from build123d import *

# Parameters (mm, degrees)
CUT_EXTRUDE_1_REACH = 23.089
SKETCH_7_R          = 1.5
CUT_EXTRUDE_2_DEPTH = 16
CUT_EXTRUDE_3_REACH = 23.089
SKETCH_8_R          = 1.5


with BuildPart() as part:
    # 草图4 → 旋转1 (revolve)
    with BuildSketch(Plane.XY, mode=Mode.PRIVATE) as revolve_1_sk:
        Polygon((0, 0), (0, 12.5), (4, 12.5), (4, 5.5), (11.5, 5.5), (11.5, 0), align=None)
    revolve(revolve_1_sk.sketch.rotate(Axis((0, 0, 0), (1, 0, 0)), 90), axis=Axis((0, 0, 0), (1, 0, 0)))

    # 草图5 → 切除-拉伸1 (cut, up to next)
    with BuildSketch(Plane(origin=(11.5, 0, 0), x_dir=(0, 0, -1), z_dir=(1, 0, 0)), mode=Mode.PRIVATE) as cut_extrude_1_sk1:
        with BuildLine():
            Line((-1.658312395, 2.5), (1.658312395, 2.5))
            ThreePointArc((1.658312395, 2.5), (0, -3), (-1.658312395, 2.5))
        make_face()
    cut_extrude_1_tool1 = extrude(cut_extrude_1_sk1.sketch, amount=-CUT_EXTRUDE_1_REACH, mode=Mode.PRIVATE) & part.part
    add(cut_extrude_1_tool1.solids().sort_by_distance((11.5, -0.111984, 0))[0], mode=Mode.SUBTRACT)

    # 草图7 → 切除-拉伸2 (cut)
    with BuildSketch(Plane(origin=(0, 6.5, 0), x_dir=(1, 0, 0), z_dir=(0, 1, 0))):
        with Locations(Location((9, 0, 0), (0, 0, 270))):
            Circle(SKETCH_7_R)
    extrude(amount=-CUT_EXTRUDE_2_DEPTH, mode=Mode.SUBTRACT)

    # 草图8 → 切除-拉伸3 (cut, up to next)
    with BuildSketch(Plane.ZY, mode=Mode.PRIVATE) as cut_extrude_3_sk1:
        with Locations((9, 0)):
            Circle(SKETCH_8_R)
    cut_extrude_3_tool1 = extrude(cut_extrude_3_sk1.sketch, amount=-CUT_EXTRUDE_3_REACH, mode=Mode.PRIVATE) & part.part
    # 草图8 → 切除-拉伸3 (cut, up to next)
    with BuildSketch(Plane.ZY, mode=Mode.PRIVATE) as cut_extrude_3_sk2:
        with Locations((0, -9)):
            Circle(SKETCH_8_R)
    cut_extrude_3_tool2 = extrude(cut_extrude_3_sk2.sketch, amount=-CUT_EXTRUDE_3_REACH, mode=Mode.PRIVATE) & part.part
    # 草图8 → 切除-拉伸3 (cut, up to next)
    with BuildSketch(Plane.ZY, mode=Mode.PRIVATE) as cut_extrude_3_sk3:
        with Locations((-9, 0)):
            Circle(SKETCH_8_R)
    cut_extrude_3_tool3 = extrude(cut_extrude_3_sk3.sketch, amount=-CUT_EXTRUDE_3_REACH, mode=Mode.PRIVATE) & part.part
    # 草图8 → 切除-拉伸3 (cut, up to next)
    with BuildSketch(Plane.ZY, mode=Mode.PRIVATE) as cut_extrude_3_sk4:
        with Locations((0, 9)):
            Circle(SKETCH_8_R)
    cut_extrude_3_tool4 = extrude(cut_extrude_3_sk4.sketch, amount=-CUT_EXTRUDE_3_REACH, mode=Mode.PRIVATE) & part.part
    add(cut_extrude_3_tool1.solids().sort_by_distance((0, 0, 9))[0], mode=Mode.SUBTRACT)
    add(cut_extrude_3_tool2.solids().sort_by_distance((0, -9, 0))[0], mode=Mode.SUBTRACT)
    add(cut_extrude_3_tool3.solids().sort_by_distance((0, 0, -9))[0], mode=Mode.SUBTRACT)
    add(cut_extrude_3_tool4.solids().sort_by_distance((0, 9, 0))[0], mode=Mode.SUBTRACT)


solid = part.part
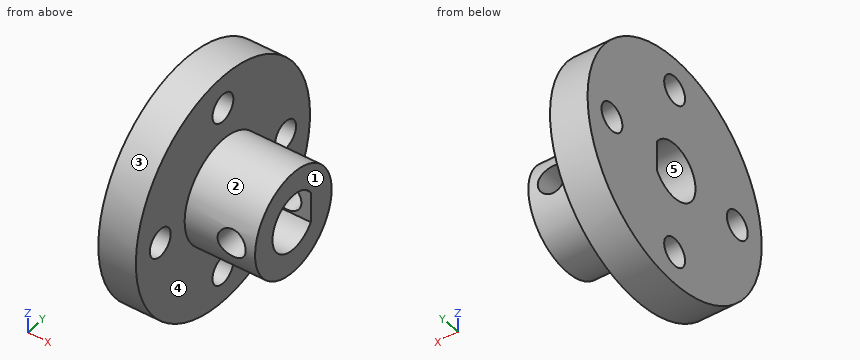
Geometry check sheet. Reference: the model listing, model coordinates, mm. Face numbers are marked on the shaded views. A direction names the side the tool comes from. Coordinates: 2 decimals unless noted, no trailing zeros. Order: outer loops, then holes, each group sorted by start corner. A loop starts at its lowest first (then second) coordinate and runs counter-clockwise, first axis right, second up. Notation, with made-up numbers: (74, -16.5) -> (88, -16.5) arc R25 cw to (88, -1.5) -> close; hole circle Ø1 at (5.25, 54). An arc over 180 degrees is marked (long way). Use a Markdown table: item, result. Add a question column.
1. Cross-section at D-D (y = -9). Enter the section's corners in (x, z), and give its area (3 significant figures).
2. Material ranges on L1, parallel to Y at x = 1.1, z = 0; L2, parallel to X at y = -10, z = -7.25; L3, parallel to Y at x = 2, z = 8, recorded low to high.
3. Go/stop test with flat-tipped pins: pin 1 Ø1.8 at (x, z) = (9, 0) entering from -Y; pin 2 Ø5 at (y, z) = (0, -9) entering from +X; pin 3 Ø3 at (x, z) = (6.5, 6.5) entering from +Y; pin 4 Ø5 at (x, z) = (9, 0) entering from -Y. Record where each tip stops, or that it passes through.
4. Cross-section at C-C (x = 2.25). Enter the section's corners in (y, z), and give its area (3 significant figures).
5. Cross-section at B-B (z = 0). Enter the section's corners in (x, y), and give its area (4 significant figures).
6. Cross-section at A-A (y = 0). Enter the section's corners in (x, z).
7. Set-up check for the marked faces 1 and 2: record each of +Z, -Z, +X, -X, +Y, -Y from which the full face is reachable in a straight line by a thin tool's end or side.
8. Mould release check, pull along Y, two halves, no side actions. Record for the marked faces 3, 4 and 5: pulls with the +Y half, pulls with the -Y half, needs draft (parallel to the pull), parting line crosses it, or undercut.
Filled sheet:
| question | item | result |
|---|---|---|
| 1 | outline | (0, -8.67) -> (4, -8.67) -> (4, -1.5) -> (0, -1.5) -> close; (0, 1.5) -> (4, 1.5) -> (4, 8.67) -> (0, 8.67) -> close |
| 1 | area | 57.4 mm2 |
| 2 | L1 | -12.5 to -10.5, -7.5 to -3, 2.5 to 7.5, 10.5 to 12.5 |
| 2 | L2 | 0 to 4 |
| 2 | L3 | -9.6 to -1.12, 1.12 to 9.6 |
| 3 | pin 1 | through |
| 3 | pin 2 | x = 4 |
| 3 | pin 3 | y = 2.29 |
| 3 | pin 4 | y = -5.5 |
| 4 | outline | circle Ø25 at (0, 0); hole circle Ø3 at (-9, 0); hole circle Ø3 at (0, -9); hole circle Ø3 at (0, 9); hole (2.5, -1.66) -> (2.5, 1.66) arc R3 ccw (long way) to start; hole circle Ø3 at (9, 0) |
| 4 | area | 435 mm2 |
| 5 | outline | (0, -12.5) -> (4, -12.5) -> (4, -10.5) -> (0, -10.5) -> close; (0, -7.5) -> (4, -7.5) -> (4, -5.5) -> (7.5, -5.5) -> (7.5, -3) -> (0, -3) -> close; (0, 2.5) -> (7.5, 2.5) -> (7.5, 5.5) -> (4, 5.5) -> (4, 7.5) -> (0, 7.5) -> close; (0, 10.5) -> (4, 10.5) -> (4, 12.5) -> (0, 12.5) -> close; (10.5, -5.5) -> (11.5, -5.5) -> (11.5, -3) -> (10.5, -3) -> close; (10.5, 2.5) -> (11.5, 2.5) -> (11.5, 5.5) -> (10.5, 5.5) -> close |
| 5 | area | 78.75 mm2 |
| 6 | outline | (0, -12.5) -> (4, -12.5) -> (4, -10.5) -> (0, -10.5) -> close; (0, -7.5) -> (4, -7.5) -> (4, -5.5) -> (11.5, -5.5) -> (11.5, -3) -> (0, -3) -> close; (0, 3) -> (11.5, 3) -> (11.5, 5.5) -> (4, 5.5) -> (4, 7.5) -> (0, 7.5) -> close; (0, 10.5) -> (4, 10.5) -> (4, 12.5) -> (0, 12.5) -> close |
| 7 | face 1 | +Z, -Z, +X, +Y, -Y |
| 7 | face 2 | +X |
| 8 | face 3 | parting line crosses it |
| 8 | face 4 | needs draft |
| 8 | face 5 | undercut |
